Job drawing, mm, ordinate dimensions from the low corner. One solid piece. Give positions to 0.01 mm unless a question says otherwise; leave off trailing zeros. Write each loop counter-clockwise with the first axis right and the second up, starting at its lowest first coordinate (ties: lowest second). Pieces come first, ordered by that corner, then holes. Notation, with made-up numbers: (17, 10.25) - (43, 10.25) arc R17 ccw to (43, 26.25) - close; hole circle Ø5 at (87.5, -27). An arc over 180 degrees is marked (long way). Answer in a Markdown table with one row per item. Add a question column.
1. Probe line 1 along Z through (x, y) = (6.75, 0.75); line 2 along X through (y, z) = (4.75, 3.25) (1 decimal); line 3 along X through (y, z) = (1, 10.5). List the from-to ranges inside material, lowest first.
2. Band-saw the part on C-C on x = 3. Write the cut outline in (y, z).
3. Band-saw the part on A-A on y = 2.75. Write the cut outline in (x, z) (1 decimal).
4. Band-saw the part on B-B on z = 4. Write the cut outline in (x, y).
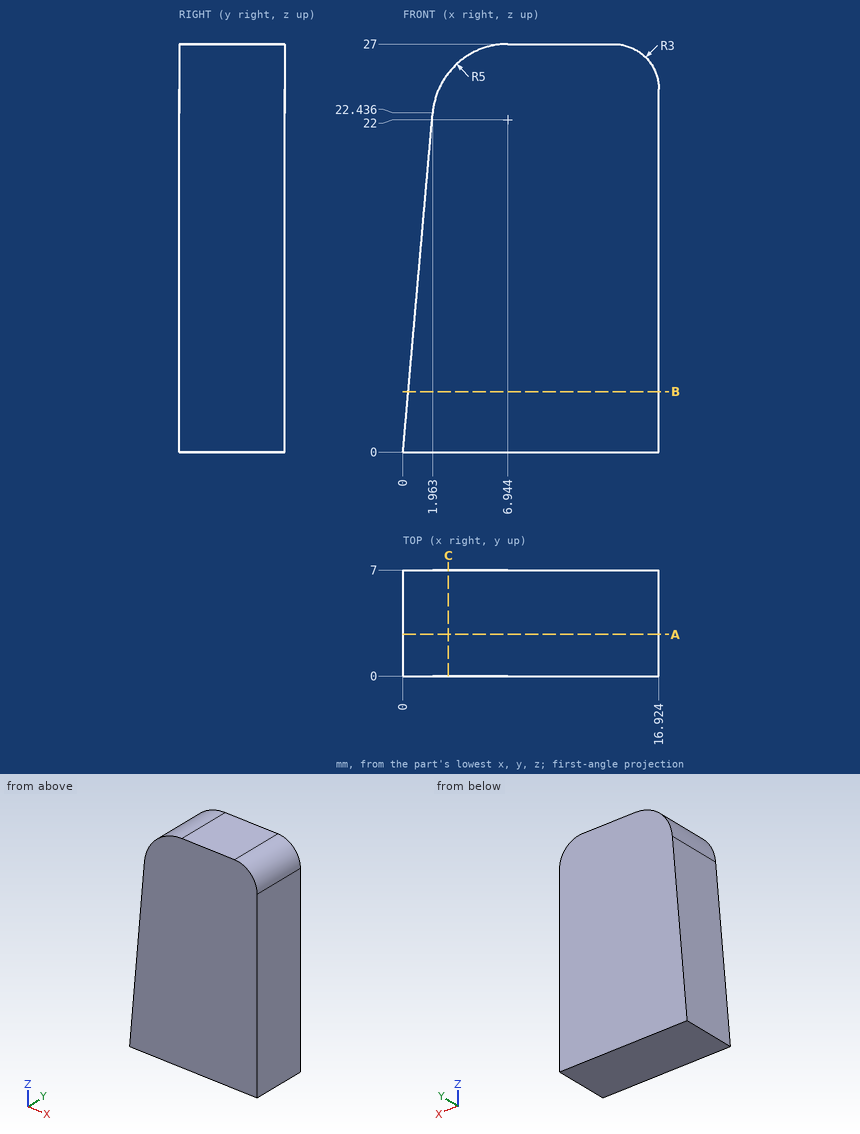
Values:
| question | item | result |
|---|---|---|
| 1 | line 1 | z = 0 to 27 |
| 1 | line 2 | x = 0.3 to 16.9 |
| 1 | line 3 | x = 0.92 to 16.92 |
| 2 | outline | (0, 0) - (7, 0) - (7, 25.07) - (0, 25.07) - close |
| 3 | outline | (0, 0) - (16.9, 0) - (16.9, 24) arc R3 ccw to (13.9, 27) - (6.9, 27) arc R5 ccw to (2, 22.4) - close |
| 4 | outline | (0.35, 0) - (16.92, 0) - (16.92, 7) - (0.35, 7) - close |
